Here's how the part is built. I have some questions about the finished solid (model axes, mm). Round coordinates to 2 decimals unless told otherwise and drop trailing zeros. Write each loop counter-clockwise with the first axis right and the second up, starting at its lowest first coordinate (ties: lowest second). Pieces come first, ordered by that corner, then holes. Notation, with made-up numbers: M 74,52 L 127,52 A28 cw 127,70 Z; hole C 71,-12.5 d2. An arc over 180 degrees is marked long. Use one line per item in the form item = value. Start each with the question number.
Q1. I'm going to push flat-ended pins straight in: pin 1 Ø11 at (x, z) = (35, 35) entering from +Y; pin 2 Ø12 at (x, z) = (-34, -14) entering from +Y. Where does each tip first touch, or does it pass through?
Q2. I want a section at A-A on z = 0. List the corners of the cut face in (x, y) for me.
Q3. I want a section at C-C on z = -35. List the corners of the cut face in (x, y) for me.
Q4. I need wall thicknesses on line 1 along Z through (x, y) = (35, -5.25); line 2 along X through (y, z) = (-7.25, 34.5); line 3 along Z through (x, y) = (0, -6). Which ranges of each line are inside material? Lowest first, please. Write a range as from..to.
Q5. I want a section at D-D on y = -3. List the corners of the cut face in (x, z) for me.
Q6. I want a section at B-B on x = 0. List the corners of the cut face in (y, z) for me, and give its area (3 significant figures).
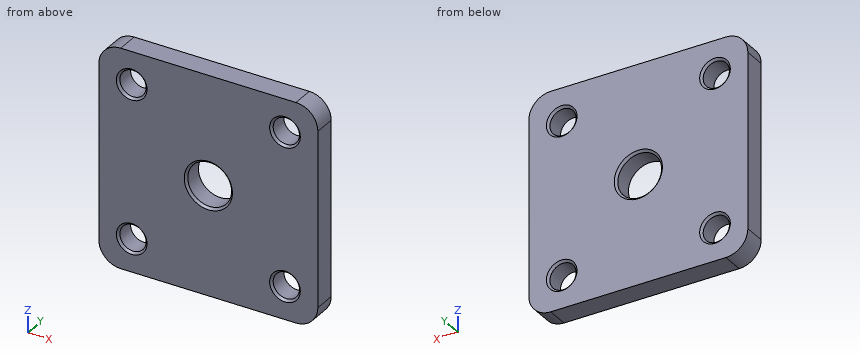
```python
from build123d import *

# Parameters (mm, degrees)
F0_W     = 100
F0_H     = 100
F0_R     = 6
F1_DEPTH = 10
F3_D     = 20
F4_R     = 10
F5_SIZE  = 1


with BuildPart() as f1:
    # F0 (on Front) → F1 (new body)
    with BuildSketch(Plane.XZ):
        Rectangle(F0_W, F0_H)
        with Locations((-35, -35)):
            Circle(F0_R, mode=Mode.SUBTRACT)
        with Locations((35, -35)):
            Circle(F0_R, mode=Mode.SUBTRACT)
        with Locations((-35, 35)):
            Circle(F0_R, mode=Mode.SUBTRACT)
        with Locations((35, 35)):
            Circle(F0_R, mode=Mode.SUBTRACT)
    extrude(amount=F1_DEPTH)

    # F3 (through all)
    with Locations(Plane.XZ.offset(10)):
        with Locations((0, 0)):
            Hole(F3_D / 2)

    # F4
    f4_edges = [f1.edges().sort_by_distance(p)[0] for p in [
        (-50, -5, -50),
        (50, -5, -50),
        (50, -5, 50),
        (-50, -5, 50),
    ]]
    fillet(f4_edges, radius=F4_R)

    # F5
    f5_edges = [f1.edges().sort_by_distance(p)[0] for p in [
        (-41, -10, 35),
        (29, -10, 35),
        (29, -10, -35),
        (-41, -10, -35),
        (-41, 0, 35),
        (-41, 0, -35),
        (29, 0, -35),
        (29, 0, 35),
        (-10, 0, 0),
        (-10, -10, 0),
    ]]
    chamfer(f5_edges, length=F5_SIZE)


solid = f1.part
```
Reported:
q1.pin_1 = through
q1.pin_2 = 0
q2.outline = M -50,-10 L -11,-10 L -10,-9 L -10,-1 L -11,0 L -50,0 Z; M 10,-9 L 11,-10 L 50,-10 L 50,0 L 11,0 L 10,-1 Z
q3.outline = M -50,-10 L -42,-10 L -41,-9 L -41,-1 L -42,0 L -50,0 Z; M -29,-9 L -28,-10 L 28,-10 L 29,-9 L 29,-1 L 28,0 L -28,0 L -29,-1 Z; M 41,-9 L 42,-10 L 50,-10 L 50,0 L 42,0 L 41,-1 Z
q4.line_1 = -50..-41, -29..29, 41..50
q4.line_2 = -50..-40.98, -29.02..29.02, 40.98..50
q4.line_3 = -50..-10, 10..50
q5.outline = M -50,-40 A10 ccw -40,-50 L 40,-50 A10 ccw 50,-40 L 50,40 A10 ccw 40,50 L -40,50 A10 ccw -50,40 Z; hole C -35,-35 d12; hole C -35,35 d12; hole C 0,0 d20; hole C 35,-35 d12; hole C 35,35 d12
q6.outline = M -10,-50 L 0,-50 L 0,-11 L -1,-10 L -9,-10 L -10,-11 Z; M -10,11 L -9,10 L -1,10 L 0,11 L 0,50 L -10,50 Z
q6.area = 798 mm^2
